The model under review builds one solid part; all positions refer to its coordinate system, in mm. Round coordinates to 2 decimals unless told otherwise and drop trailing zeros. Order: outer loops, then holes, each group sorted by start corner. A loop starts at its lowest first (then second) coordinate and runs counter-clockwise, first axis right, second up. Notation, with made-up numbers: (50.25, 78) -> (103.25, 78) arc R22 cw to (103.25, 90) -> close; hole circle Ø4 at (-9.75, -39.75). An arc over 180 degrees is marked (long way). Use a Markdown table: item, result. Add a question column.
```python
from build123d import *

# Parameters (mm, degrees)
PAD003_DEPTH = 5
SKETCH003_R  = 3.75
PAD004_DEPTH = 20
SKETCH004_R  = 3.75
PAD005_DEPTH = 7


with BuildPart() as part:
    # Sketch002 → Pad003 (new body)
    with BuildSketch(Plane.XY):
        with BuildLine():
            ThreePointArc((-19.25, 3.75), (-23, 0), (-19.25, -3.75))
            Line((-19.25, -3.75), (19.25, -3.75))
            ThreePointArc((19.25, -3.75), (23, 0), (19.25, 3.75))
            Line((-19.25, 3.75), (19.25, 3.75))
        make_face()
    extrude(amount=PAD003_DEPTH)

    # Sketch003 (on Face6 of Pad003) → Pad004 (join)
    with BuildSketch(Plane.XY.offset(5)):
        with Locations((11.5, 0)):
            Circle(SKETCH003_R)
    extrude(amount=PAD004_DEPTH)

    # Sketch004 (on Face4 of Pad004) → Pad005 (join)
    with BuildSketch(Plane(origin=(0, 0, 0), x_dir=(1, 0, 0), z_dir=(0, 0, -1))):
        with Locations((-19.25, 0)):
            Circle(SKETCH004_R)
        with Locations((19.25, 0)):
            Circle(SKETCH004_R)
    extrude(amount=PAD005_DEPTH)


solid = part.part
```
Q1. To check wall thickness, follow line 1 along Z through (x, y) = (16, 1.5); line 2 along Z through (x, y) = (10.5, -1); line 3 along X through (y, z) = (-1, 18.5). State the ranges of each line that lie inside material, in increasing order.
Q2. Add section B-B, the plane x = -6.5. Give the boundary of the cut face in (y, z).
Q3. For pin 1 (4 mm diameter, centred on x = -5.5, y = 1.5, fed in from -Z); pin 2 (4 mm diameter, centred on x = -12, z = 6, fed in from -Y); pin 3 (4 mm diameter, centred on y = 0, z = 16, fed in from -X); pin 4 (2 mm diameter, centred on x = 17, y = -1, fed in from +Z), all flat-tipped, find the tip position at first contact; note any pin that passes through.
Q4. Add section C-C, the plane z = 23.5. Give the boundary of the cut face in (x, y).
Q5. Draft analysis for pull direction X (two halves, no side actions). For faces 1 (the face through (7.754, 0.165, 14.86)), 2 (the face through (0, 0, 0)), 3 (the face through (0, 3.75, 2)), state which applies: released by +X, released by -X, zero draft, split by the parting line, or undercut.
Q6. Add section D-D, the plane y = 2.75. Give the boundary of the cut face in (x, z).
Q7. Add section A-A, the plane y = 0. Give the boundary of the cut face in (x, z).
Return value:
| question | item | result |
|---|---|---|
| 1 | line 1 | -7 to 5 |
| 1 | line 2 | 0 to 25 |
| 1 | line 3 | 7.89 to 15.11 |
| 2 | outline | (-3.75, 0) -> (3.75, 0) -> (3.75, 5) -> (-3.75, 5) -> close |
| 3 | pin 1 | z = 0 |
| 3 | pin 2 | y = -3.75 |
| 3 | pin 3 | x = 7.75 |
| 3 | pin 4 | z = 5 |
| 4 | outline | circle Ø7.5 at (11.5, 0) |
| 5 | face 1 | split by the parting line |
| 5 | face 2 | undercut |
| 5 | face 3 | zero draft |
| 6 | outline | (-21.8, -7) -> (-16.7, -7) -> (-16.7, 0) -> (16.7, 0) -> (16.7, -7) -> (21.8, -7) -> (21.8, 5) -> (14.05, 5) -> (14.05, 25) -> (8.95, 25) -> (8.95, 5) -> (-21.8, 5) -> close |
| 7 | outline | (-23, -7) -> (-15.5, -7) -> (-15.5, 0) -> (15.5, 0) -> (15.5, -7) -> (23, -7) -> (23, 5) -> (15.25, 5) -> (15.25, 25) -> (7.75, 25) -> (7.75, 5) -> (-23, 5) -> close |
